Geometry: final body of the model. Coordinates: model frame, mm. Round coordinates to 2 decimals unless told otherwise and drop trailing zeros. Use one line per item in the form item = value. Start each with the question number.
1. Pin query (flat end, axial travel): pin 1 Ø5.5 at (y, z) = (0, -38.1) entering from -X. Return the tip coordinate at first contact, or that it passes through.
2. Cut plane A-A, the plane x = 0.8. State how many separate pieces and enclosed holes the cut face has, plus the area to 3 significant figures.
3. Line query: L1, parallel to Z at x = 0.7, y = 0; L2, parallel to Y at x = 0.8, z = -126.5 (3 decimals); L3, parallel to Y at x = 0.55, z = -215.9 (1 decimal). Output: solid intervals per line, ascending.
Autodesk Inventor part; units mm, degrees
ref_plane "YZ Plane" through (0, 0, 0) normal (1, 0, 0) x (0, 1, 0)
ref_plane "XZ Plane" through (0, 0, 0) normal (0, 1, 0) x (-1, 0, 0)
ref_plane "XY Plane" through (0, 0, 0) normal (0, 0, 1) x (1, 0, 0)
sketch "main" plane through (0, 0, 0) normal (0, 0, 1) x (1, 0, 0)
  circle A0 centre (-12.3674, 169.8166) radius 2.0955
  circle A1 centre (-12.3674, 131.7166) radius 2.0955
  circle A2 centre (-12.3674, 42.8166) radius 2.0955
  circle A3 centre (-12.3674, -46.0834) radius 2.0955
  circle A4 centre (-12.3674, -134.9834) radius 2.0955
  arc A5 (6.5152, 193.7683) -> (0.3326, 201.5666) centre (0.3326, 195.2166) ccw
  line L0 (-34.5924, 159.4847) -> (-34.5924, -144.653)
  line L1 (5.8319, 198.3916) -> (44.7826, -65.1334)
  arc A6 (-34.3276, 160.7541) -> (-34.5924, 159.4847) centre (-31.4174, 159.4847) ccw
  line L2 (-34.3276, 160.7541) -> (-18.1878, 197.7554)
  line L3 (0.3326, 201.5666) -> (-12.3674, 201.5666)
  arc A7 (-12.3674, 201.5666) -> (-18.1878, 197.7554) centre (-12.3674, 195.2166) ccw
  line L4 (44.7826, -65.1334) -> (44.7826, -141.3334)
  arc A8 (-34.5924, -144.653) -> (-18.7174, -179.4334) centre (11.4451, -144.653) ccw
  line L5 (6.6826, -179.4334) -> (-18.7174, -179.4334)
  line L6 (44.7826, -141.3334) -> (6.6826, -179.4334)
  circle A9 centre (32.0826, -103.2334) radius 2.0955
  point P0 (-1.329, 35.5886)
  point P1 (-34.5924, 160.147)
  point P2 (38.4326, -84.1834)
  dimension "d0" = 12.7
  dimension "d1" = 304.8
  dimension "d2" = 15.875
  dimension "d3" = 25.4
  dimension "d4" = 3.175
  dimension "d8" = 4.191
  dimension "d9" = 4.191
  dimension "d10" = 4.191
  dimension "d11" = 4.191
  dimension "d12" = 4.191
  dimension "d13" = 4.191
sketch "Sketch1" plane through (0, 0, 0) normal (1, 0, 0) x (0, 1, 0)
  circle A0 centre (0, 0) radius 2.0955
  circle A1 centre (0, -38.1) radius 2.0955
  circle A2 centre (0, -127) radius 2.0955
  circle A3 centre (0, -215.9) radius 2.0955
  circle A4 centre (0, -304.8) radius 2.0955
  arc A5 (18.8826, 23.9517) -> (12.7, 31.75) centre (12.7, 25.4) ccw
  line L0 (-22.225, -10.3319) -> (-22.225, -314.4696)
  line L1 (18.1993, 28.575) -> (57.15, -234.95)
  arc A6 (-21.9602, -9.0625) -> (-22.225, -10.3319) centre (-19.05, -10.3319) ccw
  line L2 (-21.9602, -9.0625) -> (-5.8204, 27.9388)
  line L3 (12.7, 31.75) -> (0, 31.75)
  arc A7 (0, 31.75) -> (-5.8204, 27.9388) centre (0, 25.4) ccw
  line L4 (57.15, -234.95) -> (57.15, -311.15)
  arc A8 (-22.225, -314.4696) -> (-6.35, -349.25) centre (23.8125, -314.4696) ccw
  line L5 (19.05, -349.25) -> (-6.35, -349.25)
  line L6 (57.15, -311.15) -> (19.05, -349.25)
  circle A9 centre (44.45, -273.05) radius 2.0955
extrude "Extrusion1" add sketch "Sketch1" along normal blind 1.5875 contours L1 L4 L6 L5 A8 L0 A6 L2 A7 L3 A5
equation "\"BendRadius\" = Thickness"
equation "\"BendReliefWidth\" = Thickness"
equation "\"BendReliefDepth\" = 0.5 * Thickness"
equation "\"CornerReliefSize\" = 4 * Thickness"
equation "\"MinimumRemnant\" = 2 * Thickness"
equation "\"TransitionRadius\" = BendRadius"
equation "\"JacobiRadiusSize\" = BendRadius"
equation "\"GapSize\" = Thickness"
properties part number "Skirt" material "Acetal Resin, White"
Outcome:
q1.pin_1 = 0
q2.separate_pieces = 1
q2.enclosed_holes = 6
q2.area = 23,600 mm^2
q3.L1 = -349.25 to -306.9, -302.7 to -218, -213.8 to -129.1, -124.9 to -40.2, -36 to -2.1, 2.1 to 31.75
q3.L2 = -22.225 to -2.035, 2.035 to 41.12
q3.L3 = -22.2 to -2.1, 2.1 to 54.3
